The listing builds one solid part. Answer for the finished solid, in the listing's coordinates (mm). A direction names the side the tool comes from. Round coordinates to 2 decimals unless told otherwise and drop trailing zeros. Write each loop counter-clockwise with the first axis right and the second up, starting at its lowest first coordinate (ties: lowest second). Pieces come first, ordered by that corner, then holes.
Item 1: Find section C-C on x = 0. Give the vertices of the cut face in (y, z), then the cut area to 3 significant figures.
Item 2: Find section D-D on y = 6.5. Give the vertices of the cut face in (x, z), then the cut area to 3 significant figures.
Item 3: Find section B-B on z = -8. Give the vertices of the cut face in (x, y), then the cut area to 3 significant figures.
Item 4: A tool of negligible diameter and unlimited length cuts with its end or side. For faces 5 (the face through (0, 1.5, 4)), 6 (the face through (-15.008, 18.4, -7.9)), 7 (the face through (0, 1.5, -20)), 8 (the face through (0, 19.5, -8)), 9 (the face through (15.008, 18.4, -7.9)), from which of +Z, -Z, +X, -X, +Y, -Y can it reach the whole face along a straight path? Write none if from no direction.
Item 5: Find the intervals of material crossed by probe 1 along Y at (x, z) = (7, -8); probe 2 along Y at (x, z) = (-2, -19); probe 3 along Z at (x, y) = (-14, 7.5), in increasing order.
Item 6: Each of these flat-tipped pins is pushed along its axis until it touches: pin 1 (1 mm diameter, centred on x = -10.5, y = 10, fed in from +Z); pin 2 (9.5 mm diameter, centred on x = 2, z = 7, fed in from +Y); pin 3 (5 mm diameter, centred on y = 8.5, z = -12.5, fed in from +X). Where does it stop, or does it pass through?
Item 7: Find section A-A on y = 10.5. Give the vertices of the cut face in (x, z), then the cut area to 4 significant figures.
Item 8: For a pull along Y with two mould halves and no side action, classify faces 1 (the face through (-16, 1.5, -8)), 2 (the face through (-0.21, 3.18, -9.63)), 3 (the face through (0, 10, -17)), 4 (the face through (0, 0, -8)) as +Y half, -Y half, draft (parallel to the pull), parting line (faces both ways), or undercut.
```python
from build123d import *

# Parameters (mm, degrees)
SKETCH13_R              = 20
BOSS_EXTRUDE2_DEPTH     = 1.5
CHAMFER1_SIZE           = 2.5
ESQUISSE1_W             = 30.01666204
ESQUISSE1_H             = 18
BOSS_EXTRU_1_DEPTH      = 18
ESQUISSE2_R             = 7.5
ENL_V_MAT_EXTRU_1_DEPTH = 40


with BuildPart() as part:
    # Sketch13 → Boss-Extrude2 (new body)
    with BuildSketch(Plane(origin=(0, 0, 0), x_dir=(1, 0, 0), z_dir=(0, 1, 0))):
        with Locations(Location((0, 8, 0), (0, 0, 270))):
            Circle(SKETCH13_R)
    extrude(amount=BOSS_EXTRUDE2_DEPTH)

    # Chamfer1
    # the kernel refuses this chamfer: 2.5 mm, written as the material it takes off along each edge
    with BuildSketch(Plane(origin=(0, 1.5, -8), x_dir=(0, 0, 1), z_dir=(-1, 0, 0))) as chamfer1_piece_1:
        Polygon((20, -CHAMFER1_SIZE), (20 - CHAMFER1_SIZE, 0), (20, 0), align=None)
    revolve(axis=Axis((0, 1.5, -8), (0, 1, 0)), mode=Mode.SUBTRACT)

    # Esquisse1 → Boss.-Extru.1 (add)
    with BuildSketch(Plane(origin=(0, 1.5, 0), x_dir=(1, 0, 0), z_dir=(0, 1, 0))):
        with Locations((0, 8)):
            Rectangle(ESQUISSE1_W, ESQUISSE1_H)
    extrude(amount=BOSS_EXTRU_1_DEPTH)

    # Esquisse2 → Enlèv. mat.-Extru.1 (cut)
    with BuildSketch(Plane.ZY.offset(15.00833102)):
        with Locations((-8, 10.5)):
            Circle(ESQUISSE2_R)
    extrude(amount=-ENL_V_MAT_EXTRU_1_DEPTH, mode=Mode.SUBTRACT)


solid = part.part
```
Check values:
1. outline: (0, -27) - (1.5, -25.5) - (1.5, -17) - (19.5, -17) - (19.5, 1) - (1.5, 1) - (1.5, 9.5) - (0, 11) - close; hole circle Ø15 at (10.5, -8)
1. area: 202 mm2
2. outline: (-15.01, -17) - (15.01, -17) - (15.01, -14.34) - (-15.01, -14.34) - close; (-15.01, -1.66) - (15.01, -1.66) - (15.01, 1) - (-15.01, 1) - close
2. area: 159 mm2
3. outline: (-19, 0) - (19, 0) - (17.5, 1.5) - (15.01, 1.5) - (15.01, 3) - (-15.01, 3) - (-15.01, 1.5) - (-17.5, 1.5) - close; (-15.01, 18) - (15.01, 18) - (15.01, 19.5) - (-15.01, 19.5) - close
3. area: 145 mm2
4. face 5: +Z, +X, -X, +Y
4. face 6: +Z, -Z, -X, +Y
4. face 7: -Z, +X, -X, +Y
4. face 8: +Z, -Z, +X, -X, +Y
4. face 9: +Z, -Z, +X, +Y
5. probe 1: y = 0 to 3, 18 to 19.5
5. probe 2: y = 0 to 1.5
5. probe 3: z = -17 to -14.87, -1.13 to 1
6. pin 1: stops at z = 1
6. pin 2: stops at y = 1.5
6. pin 3: passes through
7. outline: (-15.01, -17) - (15.01, -17) - (15.01, -15.5) - (-15.01, -15.5) - close; (-15.01, -0.5) - (15.01, -0.5) - (15.01, 1) - (-15.01, 1) - close
7. area: 90.05 mm2
8. face 1: +Y half
8. face 2: undercut
8. face 3: draft
8. face 4: -Y half
